```python
from build123d import *

# Parameters (mm, degrees)
SKETCH050_W     = 56
SKETCH050_H     = 45
SKETCH050_R     = 2.5
SKETCH050_R_2   = 3.6
PAD021_DEPTH    = 5
FILLET004_R     = 5
POCKET019_DEPTH = 5
SKETCH051_R     = 1.6
PAD022_DEPTH    = 6
CHAMFER013_SIZE = 5.9999


with BuildPart() as part:
    # Sketch050 → Pad021 (new body)
    with BuildSketch(Plane.XZ):
        with Locations((-1, 25.5)):
            Rectangle(SKETCH050_W, SKETCH050_H)
        with Locations((20.3, 10)):
            Circle(SKETCH050_R, mode=Mode.SUBTRACT)
        with Locations((20.3, 41)):
            Circle(SKETCH050_R, mode=Mode.SUBTRACT)
        with Locations((-20.3, 25.5)):
            Circle(SKETCH050_R_2, mode=Mode.SUBTRACT)
    extrude(amount=PAD021_DEPTH)

    # Fillet004
    fillet004_edges = [part.edges().sort_by_distance(p)[0] for p in [
        (27, -2.5, 48),
        (27, -2.5, 3),
        (-29, -2.5, 3),
        (-29, -2.5, 48),
    ]]
    fillet(fillet004_edges, radius=FILLET004_R)

    # Sketch049 (on Face2 of Fillet004) → Pocket019 (cut)
    with BuildSketch(Plane(origin=(0, 0, 0), x_dir=(1, 0, 0), z_dir=(0, 1, 0))):
        Polygon((-7.142116, -17.15), (-7.142116, -13.85), (-10, -12.2), (-12.857884, -13.85), (-12.857884, -17.15), (-10, -18.8), align=None)
        Polygon((-7.142116, -33.85), (-10, -32.2), (-12.857884, -33.85), (-12.857884, -37.15), (-10, -38.8), (-7.142116, -37.15), align=None)
        Polygon((12.857884, -37.15), (12.857884, -33.85), (10, -32.2), (7.142116, -33.85), (7.142116, -37.15), (10, -38.8), align=None)
        Polygon((12.857884, -17.15), (12.857884, -13.85), (10, -12.2), (7.142116, -13.85), (7.142116, -17.15), (10, -18.8), align=None)
    extrude(amount=-POCKET019_DEPTH, mode=Mode.SUBTRACT)

    # Sketch051 (on Face2 of Pocket019) → Pad022 (join)
    with BuildSketch(Plane(origin=(0, 0, 0), x_dir=(1, 0, 0), z_dir=(0, 1, 0))):
        with BuildLine():
            ThreePointArc((13, -6.727386), (13.504689, -14.221819), (20, -17.994373))
            Line((20, -17.994373), (27, -17.994373))
            Line((27, -17.994373), (27, -33.005627))
            Line((20, -33.005627), (27, -33.005627))
            ThreePointArc((20, -33.005627), (13.504689, -36.778181), (13, -44.272614))
            Line((13, -44.272614), (13, -48))
            Line((-17, -48), (13, -48))
            Line((-17, -33.873171), (-17, -48))
            ThreePointArc((-17, -33.873171), (-11.3, -25.5), (-17, -17.126829))
            Line((-17, -17.126829), (-17, -3))
            Line((-17, -3), (13, -3))
            Line((13, -6.727386), (13, -3))
        make_face()
        with Locations((-10, -15.5)):
            Circle(SKETCH051_R, mode=Mode.SUBTRACT)
        with Locations((10, -15.5)):
            Circle(SKETCH051_R, mode=Mode.SUBTRACT)
        with Locations((10, -35.5)):
            Circle(SKETCH051_R, mode=Mode.SUBTRACT)
        with Locations((-10, -35.5)):
            Circle(SKETCH051_R, mode=Mode.SUBTRACT)
    extrude(amount=PAD022_DEPTH)

    # Chamfer013
    chamfer013_edges = [part.edges().sort_by_distance(p)[0] for p in [
        (-17, 0, 40.936586),
        (-17, 0, 10.063414),
        (27, 6, 25.5),
    ]]
    chamfer(chamfer013_edges, length=CHAMFER013_SIZE)


with BuildPart() as part_1:
    # Body010 placement: moved
    add(part.part.moved(Location((0, 16.5, 0))))


solid = part_1.part
```
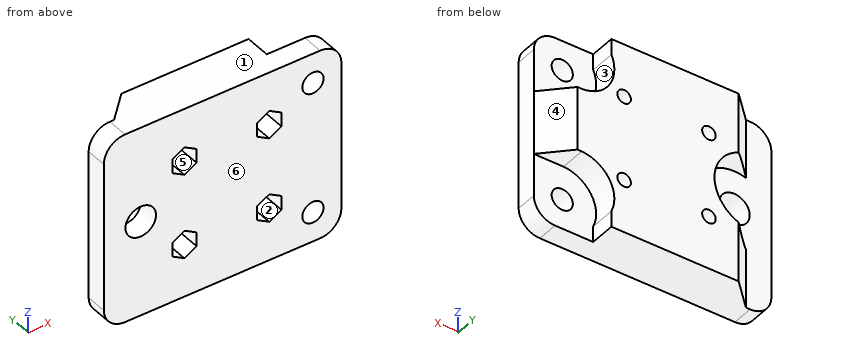
Model file for the job. Use its own axes, mm. Face numbers are marked on the shaded views. A direction names the side the tool comes from. Round coordinates to 2 decimals unless told otherwise and drop trailing zeros. Write each loop counter-clockwise with the first axis right and the second up, starting at its lowest first coordinate (ties: lowest second). Pieces come first, ordered by that corner, then holes. Notation, with made-up numbers: M 31.5,52.5 L 85.5,52.5 A8 ccw 85.5,67.5 Z; hole C -6,7 d6. An arc over 180 degrees is marked long. Put each result on its own line as item: value.
Item 1: Cut at C-C (y = 20.25). List the corners of the cut face in (x, z).
Responses:
outline: M -19.25,3 L 13,3 L 13,6.73 A8 cw 20,17.99 L 23.25,17.99 L 23.25,33.01 L 20,33.01 A8 cw 13,44.27 L 13,48 L -19.25,48 L -19.25,34.44 A9 cw -19.25,16.56 Z; hole C -10,15.5 d3.2; hole C -10,35.5 d3.2; hole C 10,15.5 d3.2; hole C 10,35.5 d3.2
Item 2: Tool access for the marked faces 1, 2 and 3: list every direction of +Z, -Z, +X, -X, +Y, -Y with a clear straight run to the whole face (end or side of a thin tool).
Responses:
face 1: +Z, +X, -X, +Y, -Y
face 2: -Y
face 3: +X, +Y
Item 3: Mould opens along X. For the marked faces 4, 5 and 6 say: +X half, -X half, draft (parallel to the pull), parting line (faces both ways), or undercut.
Responses:
face 4: +X half
face 5: undercut
face 6: draft
Item 4: Flat gauge pins, fed straight in: P1, Ø4, axis at x = -21, z = 33, coming from the +Y side; P2, Ø20.5, axis at x = -20.3, z = 25.5, coming from the +Y side; P3, Ø6.5, axis at x = -20.3, z = 25.5, coming from the -Y side; P4, Ø3, axis at x = 11, z = 35, coming from the -Y side. Where does each tip first touch, or does it go through?
Responses:
P1: y = 19.85
P2: y = 22.5
P3: through
P4: y = 16.5
Item 5: Cut at D-D (x = -9). List the corners of the cut face in (y, z), and give its area (3 significant figures).
Responses:
outline: M 11.5,3 L 22.5,3 L 22.5,14.25 L 16.5,14.25 L 16.5,12.78 L 11.5,12.78 Z; M 11.5,18.22 L 16.5,18.22 L 16.5,16.75 L 22.5,16.75 L 22.5,34.25 L 16.5,34.25 L 16.5,32.78 L 11.5,32.78 Z; M 11.5,38.22 L 16.5,38.22 L 16.5,36.75 L 22.5,36.75 L 22.5,48 L 11.5,48 Z
area: 411 mm²
Item 6: Cut at B-B (z = 15.5). State how many separate pieces and enclosed holes the cut face has, and give its area (3 significant figures).
Responses:
separate pieces: 3
enclosed holes: 0
area: 391 mm²
Item 7: Probe L1, parallel to Z at x = 10, y = 18.95; L2, parallel to Z at x = 20.3, y = 12.8; L3, parallel to X at y = 19, z = 35.5. List the from-to ranges inside material, lowest first. Write a range as from..to.
Responses:
L1: 3..13.9, 17.1..33.9, 37.1..48
L2: 3..7.5, 12.5..38.5, 43.5..48
L3: -20.5..-11.6, -8.4..8.4, 11.6..14.49
